from build123d import *

# Parameters (mm, degrees)
SKETCH1_R           = 5
SKETCH1_R_2         = 15
BOSS_EXTRUDE1_DEPTH = 5


with BuildPart() as part:
    # Sketch1 → Boss-Extrude1 (new body)
    with BuildSketch(Plane.XY):
        with BuildLine():
            Line((0, 25.040916558), (-175.857142857, 14.97549018))
            ThreePointArc((-175.857142857, 14.97549018), (-190, 0), (-175.857142857, -14.97549018))
            Line((-175.857142857, -14.97549018), (0, -25.040916558))
            Line((0, -25.040916558), (175.857142857, -14.97549018))
            ThreePointArc((175.857142857, -14.97549018), (190, 0), (175.857142857, 14.97549018))
            Line((175.857142857, 14.97549018), (0, 25.040916558))
        make_face()
        with Locations((-175, 0)):
            Circle(SKETCH1_R, mode=Mode.SUBTRACT)
        Circle(SKETCH1_R_2, mode=Mode.SUBTRACT)
        with Locations((175, 0)):
            Circle(SKETCH1_R, mode=Mode.SUBTRACT)
    extrude(amount=BOSS_EXTRUDE1_DEPTH)


solid = part.part
Design review of the part built by this model. Coordinates are the model's own, in mm. Give positions to 0.01 mm unless a question says otherwise; leave off trailing zeros. Order: outer loops, then holes, each group sorted by start corner. A loop starts at its lowest first (then second) coordinate and runs counter-clockwise, first axis right, second up. Notation, with made-up numbers: (-36, 77.5) - (20, 77.5) arc R29 ccw to (20, 104.5) - close; hole circle Ø11 at (-25, 75.25). An arc over 180 degrees is marked (long way). Use CSV: the item, a comma, the result in double quotes. Start each with the question number.
Q1. Take a section at B-B (z = 2.55). State the section outline as (x, y) points.
Q2. Draft analysis for pull direction X (two halves, no side actions). For faces 1 (the face through (-14.985, 0.66, 2.465)), 2 (the face through (-86.7, 20.08, 2.46)), 3 (the face through (86.7, -20.08, 2.46)), state which applies: pulls with the +X half, pulls with the -X half, needs draft (parallel to the pull), parting line crosses it, or undercut.
Q3. For line 1 (Y direction, x = 175, z = 1.75); line 2 (X direction, y = 7, z = 2); line 3 (X direction, y = -7.5, z = 1.55), list the stretches that pass through material, from the lowest coordinate up.
Q4. Take a section at D-D (x = 108). State the section outline as (y, z) points.
Q5. For P1, Ø1.5, axis at x = 127, z = 2, coming from the -Y side; P2, Ø3, axis at x = 131.5, z = 3.5, coming from the +Y side; P3, Ø1, axis at x = 105.5, z = 2.5, coming from the -Y side, all flat-tipped, find the tip position at first contact; note any pin that passes through.
Q6. Take a section at A-A (y = 0). State the section outline as (x, z) points.
Q7. Take a section at C-C (x = -92). State the section outline as (y, z) points, and give its area (3 significant figures).
Calculated:
1,outline,"(-175.86, -14.98) - (0, -25.04) - (175.86, -14.98) arc R15 ccw to (175.86, 14.98) - (0, 25.04) - (-175.86, 14.98) arc R15 ccw to start; hole circle Ø10 at (-175, 0); hole circle Ø30 at (0, 0); hole circle Ø10 at (175, 0)"
2,face 1,"undercut"
2,face 2,"pulls with the -X half"
2,face 3,"pulls with the +X half"
3,line 1,"y = -15.02 to -5, 5 to 15.02"
3,line 2,"x = -188.27 to -13.27, 13.27 to 188.27"
3,line 3,"x = -187.99 to -12.99, 12.99 to 187.99"
4,outline,"(-18.86, 0) - (18.86, 0) - (18.86, 5) - (-18.86, 5) - close"
5,P1,"stops at y = -17.81"
5,P2,"stops at y = 17.6"
5,P3,"stops at y = -19.03"
6,outline,"(-190, 0) - (-180, 0) - (-180, 5) - (-190, 5) - close; (-170, 0) - (-15, 0) - (-15, 5) - (-170, 5) - close; (15, 0) - (170, 0) - (170, 5) - (15, 5) - close; (180, 0) - (190, 0) - (190, 5) - (180, 5) - close"
7,outline,"(-19.78, 0) - (19.78, 0) - (19.78, 5) - (-19.78, 5) - close"
7,area,"198 mm²"
